from build123d import *

# Parameters (mm, degrees)
BOSS_EXTRUDE1_DEPTH     = 250
BOSS_EXTRUDE2_START     = -20
BOSS_EXTRUDE2_OUTLINE_W = 15
BOSS_EXTRUDE2_OUTLINE_H = 20
BOSS_EXTRUDE2_DEPTH     = 20
BOSS_EXTRUDE3_START     = -20
BOSS_EXTRUDE3_OUTLINE_W = 15
BOSS_EXTRUDE3_OUTLINE_H = 20
BOSS_EXTRUDE3_DEPTH     = 20
SKETCH8_W               = 15
SKETCH8_H               = 20
BOSS_EXTRUDE5_DEPTH     = 20
SKETCH9_W               = 15
SKETCH9_H               = 20
BOSS_EXTRUDE6_DEPTH     = 20
SKETCH11_R              = 2
CUT_EXTRUDE1_DEPTH      = 10
SKETCH12_R              = 5
CUT_EXTRUDE2_DEPTH      = 10
CUT_EXTRUDE3_START      = -10
SKETCH13_R              = 5
CUT_EXTRUDE3_DEPTH      = 10


# Read off the part's stored shape, not the designer's step: Boss-Extrude2, Boss-Extrude3
with BuildPart() as part:
    # Sketch1 → Boss-Extrude1 (new body)
    with BuildSketch(Plane(origin=(0, 0, 0), x_dir=(1, 0, 0), z_dir=(0, 1, 0))):
        with BuildLine():
            Line((-10, 30), (-10, 200))
            ThreePointArc((-10, 200), (1.715728753, 228.284271247), (30, 240))
            Line((30, 240), (190, 240))
            ThreePointArc((190, 240), (218.284271247, 228.284271247), (230, 200))
            Line((230, 200), (230, 30))
            ThreePointArc((230, 30), (218.284271247, 1.715728753), (190, -10))
            Line((190, -10), (30, -10))
            ThreePointArc((30, -10), (1.715728753, 1.715728753), (-10, 30))
        make_face()
        with BuildLine():
            Line((30, 0), (190, 0))
            ThreePointArc((190, 0), (211.213203436, 8.786796564), (220, 30))
            Line((220, 30), (220, 200))
            ThreePointArc((220, 200), (211.213203436, 221.213203436), (190, 230))
            Line((190, 230), (30, 230))
            ThreePointArc((30, 230), (8.786796564, 221.213203436), (0, 200))
            Line((0, 200), (0, 30))
            ThreePointArc((0, 30), (8.786796564, 8.786796564), (30, 0))
        make_face(mode=Mode.SUBTRACT)
    extrude(amount=BOSS_EXTRUDE1_DEPTH)

    # Boss-Extrude2 outline → Boss-Extrude2 (add)
    with BuildSketch(Plane.ZY.offset(10).offset(BOSS_EXTRUDE2_START)):
        with Locations((-192.5, 10)):
            Rectangle(BOSS_EXTRUDE2_OUTLINE_W, BOSS_EXTRUDE2_OUTLINE_H)
        with Locations((-12.5, 10)):
            Rectangle(BOSS_EXTRUDE2_OUTLINE_W, BOSS_EXTRUDE2_OUTLINE_H)
        with Locations((-42.5, 10)):
            Rectangle(BOSS_EXTRUDE2_OUTLINE_W, BOSS_EXTRUDE2_OUTLINE_H)
        with Locations((-72.5, 10)):
            Rectangle(BOSS_EXTRUDE2_OUTLINE_W, BOSS_EXTRUDE2_OUTLINE_H)
        with Locations((-102.5, 10)):
            Rectangle(BOSS_EXTRUDE2_OUTLINE_W, BOSS_EXTRUDE2_OUTLINE_H)
        with Locations((-132.5, 10)):
            Rectangle(BOSS_EXTRUDE2_OUTLINE_W, BOSS_EXTRUDE2_OUTLINE_H)
        with Locations((-162.5, 10)):
            Rectangle(BOSS_EXTRUDE2_OUTLINE_W, BOSS_EXTRUDE2_OUTLINE_H)
    extrude(amount=BOSS_EXTRUDE2_DEPTH)

    # Boss-Extrude3 outline → Boss-Extrude3 (add)
    with BuildSketch(Plane(origin=(230, 0, 0), x_dir=(0, 0, -1), z_dir=(1, 0, 0)).offset(BOSS_EXTRUDE3_START)):
        with Locations((192.5, 10)):
            Rectangle(BOSS_EXTRUDE3_OUTLINE_W, BOSS_EXTRUDE3_OUTLINE_H)
        with Locations((12.5, 10)):
            Rectangle(BOSS_EXTRUDE3_OUTLINE_W, BOSS_EXTRUDE3_OUTLINE_H)
        with Locations((42.5, 10)):
            Rectangle(BOSS_EXTRUDE3_OUTLINE_W, BOSS_EXTRUDE3_OUTLINE_H)
        with Locations((72.5, 10)):
            Rectangle(BOSS_EXTRUDE3_OUTLINE_W, BOSS_EXTRUDE3_OUTLINE_H)
        with Locations((102.5, 10)):
            Rectangle(BOSS_EXTRUDE3_OUTLINE_W, BOSS_EXTRUDE3_OUTLINE_H)
        with Locations((132.5, 10)):
            Rectangle(BOSS_EXTRUDE3_OUTLINE_W, BOSS_EXTRUDE3_OUTLINE_H)
        with Locations((162.5, 10)):
            Rectangle(BOSS_EXTRUDE3_OUTLINE_W, BOSS_EXTRUDE3_OUTLINE_H)
    extrude(amount=BOSS_EXTRUDE3_DEPTH)

    # Sketch8 → Boss-Extrude5 (add)
    with BuildSketch(Plane(origin=(-10, 0, 0), x_dir=(0, 0, -1), z_dir=(1, 0, 0))):
        with Locations((172.5, 240)):
            Rectangle(SKETCH8_W, SKETCH8_H)
        with Locations((142.5, 240)):
            Rectangle(SKETCH8_W, SKETCH8_H)
        with Locations((112.5, 240)):
            Rectangle(SKETCH8_W, SKETCH8_H)
        with Locations((52.5, 240)):
            Rectangle(SKETCH8_W, SKETCH8_H)
        with Locations((232.5, 240)):
            Rectangle(SKETCH8_W, SKETCH8_H)
        with Locations((82.5, 240)):
            Rectangle(SKETCH8_W, SKETCH8_H)
        with Locations((202.5, 240)):
            Rectangle(SKETCH8_W, SKETCH8_H)
    extrude(amount=BOSS_EXTRUDE5_DEPTH)

    # Sketch9 → Boss-Extrude6 (add)
    with BuildSketch(Plane(origin=(230, 0, 0), x_dir=(0, 0, -1), z_dir=(1, 0, 0))):
        with Locations((82.5, 240)):
            Rectangle(SKETCH9_W, SKETCH9_H)
        with Locations((142.5, 240)):
            Rectangle(SKETCH9_W, SKETCH9_H)
        with Locations((172.5, 240)):
            Rectangle(SKETCH9_W, SKETCH9_H)
        with Locations((52.5, 240)):
            Rectangle(SKETCH9_W, SKETCH9_H)
        with Locations((112.5, 240)):
            Rectangle(SKETCH9_W, SKETCH9_H)
        with Locations((202.5, 240)):
            Rectangle(SKETCH9_W, SKETCH9_H)
        with Locations((232.5, 240)):
            Rectangle(SKETCH9_W, SKETCH9_H)
    extrude(amount=-BOSS_EXTRUDE6_DEPTH)

    # Sketch11 → Cut-Extrude1 (cut)
    with BuildSketch(Plane(origin=(230, 0, 0), x_dir=(0, 0, -1), z_dir=(1, 0, 0))):
        with Locations((78, 196.104898216)):
            Circle(SKETCH11_R)
        with Locations(Location((78, 126.104898216, 0), (0, 0, 180))):
            Circle(SKETCH11_R)
        with Locations((162, 126.104898216)):
            Circle(SKETCH11_R)
        with Locations(Location((162, 196.104898216, 0), (0, 0, 180))):
            Circle(SKETCH11_R)
    extrude(amount=-CUT_EXTRUDE1_DEPTH, mode=Mode.SUBTRACT)

    # Sketch12 → Cut-Extrude2 (cut)
    with BuildSketch(Plane(origin=(0, 0, -240), x_dir=(-1, 0, 0), z_dir=(0, 0, -1))):
        with Locations((-150, 240)):
            Circle(SKETCH12_R)
        with Locations(Location((-70, 240, 0), (0, 0, 180))):
            Circle(SKETCH12_R)
        with Locations((-70, 10)):
            Circle(SKETCH12_R)
        with Locations(Location((-150, 10, 0), (0, 0, 180))):
            Circle(SKETCH12_R)
    extrude(amount=-CUT_EXTRUDE2_DEPTH, mode=Mode.SUBTRACT)

    # Sketch13 → Cut-Extrude3 (cut)
    with BuildSketch(Plane.XY.offset(10).offset(CUT_EXTRUDE3_START)):
        with Locations((70, 240)):
            Circle(SKETCH13_R)
        with Locations(Location((150, 240, 0), (0, 0, 180))):
            Circle(SKETCH13_R)
        with Locations((150, 10)):
            Circle(SKETCH13_R)
        with Locations(Location((70, 10, 0), (0, 0, 180))):
            Circle(SKETCH13_R)
    extrude(amount=CUT_EXTRUDE3_DEPTH, mode=Mode.SUBTRACT)


solid = part.part
Verification items for the finished model (mm, model axes). A direction names the side the tool comes from. Coordinates: 2 decimals unless noted, no trailing zeros. Loops run counter-clockwise (first coordinate to the right, second up) from the corner with the lowest first, then second, coordinate; pieces in that order, holes last. Notation, with made-up numbers: M 63,10.25 L 99,10.25 A33 ccw 99,41.25 Z; hole C 9.5,27 d2. An arc over 180 degrees is marked long. One line per item, written item: value.
1. Section check C-C on y = 132.5. Record the cut outline in (x, z).
Answers follow:
outline: M -10,-200 A40 ccw 30,-240 L 190,-240 A40 ccw 230,-200 L 230,-30 A40 ccw 190,10 L 30,10 A40 ccw -10,-30 Z; hole M 0,-200 A30 ccw 30,-230 L 190,-230 A30 ccw 220,-200 L 220,-30 A30 ccw 190,0 L 30,0 A30 ccw 0,-30 Z
2. Mould release check, pull along Y, two halves, no side actions. Record for faces 1 (the cylindrical face through (145, 10, 5)), 2 (the flat face through (215, 10, -95)): pulls with the +Y half, pulls with the -Y half, needs draft (parallel to the pull), parting line crosses it, or undercut.
Answers follow:
face 1: undercut
face 2: needs draft
3. Material ranges on line 1 along Y through (x, z) = (150, 6); line 2 along X through (y, z) = (76.5, -87); line 3 along Z through (x, y) = (159, 124), recorded low to high. Write a range as from..to.
Answers follow:
line 1: 0..5, 15..235, 245..250
line 2: -10..0, 220..230
line 3: -240..-230, 0..10
4. Section check D-D on z = -215.5. Record the cut outline in (x, y), plus the area to 3 significant figures.
Answers follow:
outline: M -6.87,0 L 4.31,0 L 4.31,250 L -6.87,250 Z; M 215.69,0 L 226.87,0 L 226.87,250 L 215.69,250 Z
area: 5,590 mm^2
5. Section check A-A on x = 150. Record the cut outline in (y, z), plus the area to 3 significant figures.
Answers follow:
outline: M 0,-240 L 5,-240 L 5,-230 L 0,-230 Z; M 0,0 L 5,0 L 5,10 L 0,10 Z; M 15,-240 L 235,-240 L 235,-230 L 15,-230 Z; M 15,0 L 235,0 L 235,10 L 15,10 Z; M 245,-240 L 250,-240 L 250,-230 L 245,-230 Z; M 245,0 L 250,0 L 250,10 L 245,10 Z
area: 4,600 mm^2
6. Section check B-B on x = 106. Record the cut outline in (y, z), plus the area to 3 significant figures.
Answers follow:
outline: M 0,-240 L 250,-240 L 250,-230 L 0,-230 Z; M 0,0 L 250,0 L 250,10 L 0,10 Z
area: 5,000 mm^2
7. Set-up check for faces 3 (the cylindrical face through (211.445, 123.25, -220.979)), 4 (the flat face through (5, 10, -95)), 5 (the flat face through (215, 230, -202)): record each of +Z, -Z, +X, -X, +Y, -Y from which the full face is reachable in a straight line by a thin tool's end or side.
Answers follow:
face 3: -Y
face 4: +Y, -Y
face 5: none
8. Gauge pin test, flat ends, axial feed: P1, Ø5, axis at x = 215.5, y = 10.5, coming from the +Z side; P2, Ø11, axis at x = 215.5, y = 236.5, coming from the +Z side; P3, Ø8, axis at x = 6.5, y = 12.5, coming from the -Z side; P4, Ø16, axis at x = 150, y = 240, coming from the +Z side. Record the tip position at first contact, or that the pin passes through.
Answers follow:
P1: z = 2.73
P2: z = 4.64
P3: z = -234.92
P4: z = 10
